from build123d import *

# Parameters (mm, degrees)
F0_W     = 150
F0_H     = 150
F1_DEPTH = 9
F2_R     = 3
F3_DEPTH = 9.001
F4_R     = 1.5
F5_DEPTH = 9.001
F6_R     = 3
F7_DEPTH = 3


with BuildPart() as f1:
    # F0 (on Top) → F1 (new body)
    with BuildSketch(Plane.XY):
        with Locations((-74.065436, -102.650428)):
            Rectangle(F0_W, F0_H)
    extrude(amount=F1_DEPTH)

    # F2 (on face) → F3 (cut, through all)
    with BuildSketch(Plane.XY.offset(9)):
        with Locations((-124.065436, -52.650428)):
            Circle(F2_R)
        with Locations((-124.065436, -152.650428)):
            Circle(F2_R)
        with Locations((-24.065436, -152.650428)):
            Circle(F2_R)
        with Locations((-24.065436, -52.650428)):
            Circle(F2_R)
    extrude(amount=-F3_DEPTH, mode=Mode.SUBTRACT)

    # F4 (on face) → F5 (cut, through all)
    with BuildSketch(Plane(origin=(0, 0, 0), x_dir=(1, 0, 0), z_dir=(0, 0, -1))):
        with Locations((-144.565436, 173.150428)):
            Circle(F4_R)
        with Locations((-74.065436, 173.150428)):
            Circle(F4_R)
        with Locations((-3.565436, 173.150428)):
            Circle(F4_R)
        with Locations((-3.565436, 102.650428)):
            Circle(F4_R)
        with Locations((-3.565436, 32.150428)):
            Circle(F4_R)
        with Locations((-74.065436, 32.150428)):
            Circle(F4_R)
        with Locations((-144.565436, 32.150428)):
            Circle(F4_R)
        with Locations((-144.565436, 102.650428)):
            Circle(F4_R)
        with Locations((-74.065436, 102.650428)):
            Circle(F4_R)
    extrude(amount=-F5_DEPTH, mode=Mode.SUBTRACT)

    # F6 (on face) → F7 (cut)
    with BuildSketch(Plane(origin=(0, 0, 0), x_dir=(1, 0, 0), z_dir=(0, 0, -1))):
        with Locations((-144.565436, 173.150428)):
            Circle(F6_R)
        with Locations((-74.065436, 173.150428)):
            Circle(F6_R)
        with Locations((-3.565436, 173.150428)):
            Circle(F6_R)
        with Locations((-3.565436, 102.650428)):
            Circle(F6_R)
        with Locations((-74.065436, 102.650428)):
            Circle(F6_R)
        with Locations((-144.565436, 102.650428)):
            Circle(F6_R)
        with Locations((-144.565436, 32.150428)):
            Circle(F6_R)
        with Locations((-74.065436, 32.150428)):
            Circle(F6_R)
        with Locations((-3.565436, 32.150428)):
            Circle(F6_R)
    extrude(amount=-F7_DEPTH, mode=Mode.SUBTRACT)


solid = f1.part
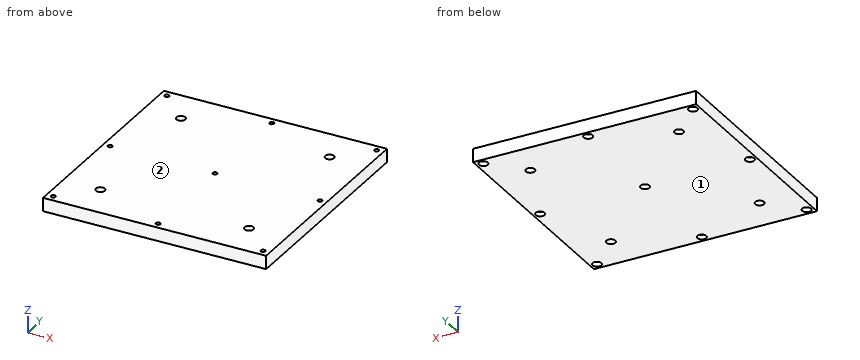
Geometry: final body of the model. Coordinates: model frame, mm. Face numbers are marked on the shaded views. Give positions to 0.01 mm unless a question says otherwise; leave off trailing zeros. Answer as CSV lines item,"result". Start each with the question number.
1. Draft query along Z for the marked faces 1 and 2. Return one class per face: released by +Z, released by -Z, zero draft, split by the parting line, or undercut.
2. Ray query, L1, parallel to X at y = -170.5, z = 1.75; L2, parallel to X at y = -155, z = 5.75. Return the intervals inside material, ascending.
3. Pin query (flat end, axial travel): P1, Ø5, axis at x = -144.57, y = -102.65, coming from the -Z side. Return the tip coordinate at first contact, or that it passes through.
Answers:
1,face 1,"released by -Z"
1,face 2,"released by +Z"
2,L1,"x = -149.07 to -145.97, -143.16 to -75.47, -72.66 to -4.97, -2.16 to 0.93"
2,L2,"x = -149.07 to -125.93, -122.2 to -25.93, -22.2 to 0.93"
3,P1,"stops at z = 3"
